Geometry check sheet. Reference: drawing and pictorial views, mm from the part's lowest x, y, z. Give positions to 0.01 mm unless a question says otherwise; leave off trailing zeros. Loops run counter-clockwise (first coordinate to the right, second up) from the corner with the lowest first, then second, coordinate; pieces in that order, holes last. Notation, with made-up numbers: (-30.75, 21) - (10.25, 21) arc R14 ccw to (10.25, 29) - close; hole circle Ø4 at (-2, -2). An arc over 180 degrees is marked (long way). One line per question, with ' | ' between items. Start each with the question number.
1. Section check C-C, the plane z = 3.5. Enter the section's corners in (x, y).
2. Mould release check, pull along X, two halves, no side actions. Record for the marked faces 1, 2, 3 and 4: +X half, -X half, draft (parallel to the pull), parting line (faces both ways), or undercut.
3. Thickness scan on line 1 along X through (y, z) = (26.5, 6.25); line 2 along X through (y, z) = (32, 3.5); line 3 along Y through (x, z) = (8.5, 0.75) (1 decimal). Record the ranges inside material, lowest first. Write a range as from..to.
4. Section check D-D, the plane y = 9. Enter the section's corners in (x, z).
5. Depth check by flat-ended pin: pin 1 Ø1 at (y, z) = (47.5, 4.5) entering from +X; pin 2 Ø1.5 at (x, z) = (7.5, 4) entering from +Y. Enter the tip coordinate at first touch or a pass-through.
6. Section check A-A, the plane x = 14. Enter the section's corners in (y, z), then the cut area to 3 significant figures.
7. Section check B-B, the plane y = 15.5. Enter the section's corners in (x, z).
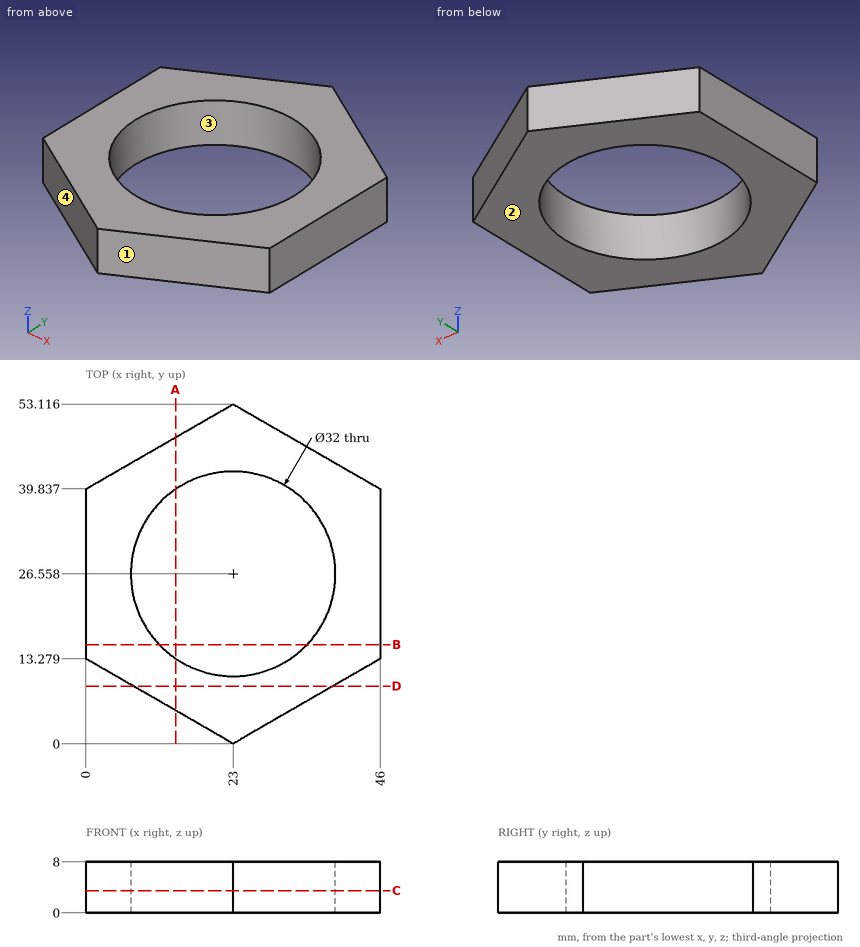
Results list:
1) outline: (0, 13.28) - (23, 0) - (46, 13.28) - (46, 39.84) - (23, 53.12) - (0, 39.84) - close; hole circle Ø32 at (23, 26.56)
2) face 1: +X half | face 2: draft | face 3: undercut | face 4: -X half
3) line 1: 0..7, 39..46 | line 2: 0..7.95, 38.05..46 | line 3: 8.4..19.8, 33.3..44.7
4) outline: (7.41, 0) - (38.59, 0) - (38.59, 8) - (7.41, 8) - close
5) pin 1: x = 33.59 | pin 2: y = 44.6
6) outline: (5.2, 0) - (13.33, 0) - (13.33, 8) - (5.2, 8) - close; (39.79, 0) - (47.92, 0) - (47.92, 8) - (39.79, 8) - close | area: 130 mm²
7) outline: (0, 0) - (11.44, 0) - (11.44, 8) - (0, 8) - close; (34.56, 0) - (46, 0) - (46, 8) - (34.56, 8) - close
